```python
from build123d import *

# Parameters (mm, degrees)
F0_W     = 19
F0_H     = 19
F0_W_2   = 13.5
F0_H_2   = 13.5
F1_DEPTH = 12.5
F2_W     = 25
F2_H     = 34
F3_DEPTH = 2.5
F4_W     = 25
F4_H     = 2
F5_DEPTH = 30
F6_W     = 2
F6_H     = 25
F7_DEPTH = 20
F8_W     = 32.5
F8_H     = 10
F9_DEPTH = 2


with BuildPart() as f1:
    # F0 (on Front) → F1 (new body, symmetric)
    with BuildSketch(Plane.XZ):
        Rectangle(F0_W, F0_H)
        Rectangle(F0_W_2, F0_H_2, mode=Mode.SUBTRACT)
    extrude(amount=F1_DEPTH, both=True)

    # F2 (on face) → F3 (join)
    with BuildSketch(Plane(origin=(-9.5, 0, 0), x_dir=(0, -1, 0), z_dir=(-1, 0, 0))):
        with Locations((0, -7.5)):
            Rectangle(F2_W, F2_H)
    extrude(amount=-F3_DEPTH)

    # F4 (on face) → F5 (join)
    with BuildSketch(Plane(origin=(-9.5, 0, 0), x_dir=(0, -1, 0), z_dir=(-1, 0, 0))):
        with Locations((0, -23.5)):
            Rectangle(F4_W, F4_H)
    extrude(amount=F5_DEPTH)

    # F6 (on face) → F7 (join)
    with BuildSketch(Plane.XY.offset(-22.5)):
        with Locations((-38.5, 0)):
            Rectangle(F6_W, F6_H)
    extrude(amount=F7_DEPTH)

    # F8 (on face) → F9 (join)
    with BuildSketch(Plane(origin=(0, 12.5, 0), x_dir=(-1, 0, 0), z_dir=(0, 1, 0))):
        with Locations((23.25, -19.5)):
            Rectangle(F8_W, F8_H)
    extrude(amount=-F9_DEPTH)


solid = f1.part
```
Design review of the part built by this model. Coordinates are the model's own, in mm. A direction names the side the tool comes from. Coordinates: 2 decimals unless noted, no trailing zeros. Order: outer loops, then holes, each group sorted by start corner. A loop starts at its lowest first (then second) coordinate and runs counter-clockwise, first axis right, second up. Notation, with made-up numbers: (34, 20.25) - (41, 20.25) arc R34 ccw to (41, 58.25) - close; hole circle Ø1 at (-17, 41.25). An arc over 180 degrees is marked (long way). One line per question, with ' | ' between items.
Q1. To check wall thickness, follow line 1 along X through (y, z) = (-7.25, -5); line 2 along X through (y, z) = (8, -18); line 3 along X through (y, z) = (-10.75, -2). State the ranges of each line that lie inside material, in increasing order.
Answer key:
line 1: x = -39.5 to -37.5, -9.5 to -6.75, 6.75 to 9.5 | line 2: x = -39.5 to -37.5, -9.5 to -7 | line 3: x = -9.5 to -6.75, 6.75 to 9.5
Q2. For faces 1 (the flat face through (6.75, 0, 0)), 2 (the flat face through (-23, 12, -14.5)), 3 (the flat face through (-23, -1, -22.5)), 4 (the flat face through (-39, 0, -2.5)), 5 (the flat face through (1, 0, -9.5)), list the 3-axis set-ups (+Z, -Z, +X, -X, +Y, -Y) from which the entire face can be reached by the end or side of a thin tool; tool diameter is ignored.
Answer key:
face 1: +Y, -Y | face 2: +Z, +Y, -Y | face 3: +Z, -Y | face 4: +Z, -X, +Y, -Y | face 5: -Z, +X, +Y, -Y
Q3. Consider section C-C, the plane y = 0.75. Give the boundary of the cut face in (x, z), then the cut area to 3 significant figures.
Answer key:
outline: (-39.5, -24.5) - (-7, -24.5) - (-7, -9.5) - (9.5, -9.5) - (9.5, 9.5) - (-9.5, 9.5) - (-9.5, -22.5) - (-37.5, -22.5) - (-37.5, -2.5) - (-39.5, -2.5) - close; hole (-6.75, -6.75) - (6.75, -6.75) - (6.75, 6.75) - (-6.75, 6.75) - close | area: 316 mm2
Q4. Consider section A-A, the plane z = -1. Give the boundary of the cut face in (x, y), then the cut area to 4 significant figures.
Answer key:
outline: (-9.5, -12.5) - (-6.75, -12.5) - (-6.75, 12.5) - (-9.5, 12.5) - close; (6.75, -12.5) - (9.5, -12.5) - (9.5, 12.5) - (6.75, 12.5) - close | area: 137.5 mm2
Q5. Clearance check with flat-ended pins moving along their axes: pin 1 Ø8 at (y, z) = (0.5, 0) entering from -X; pin 2 Ø11.5 at (x, y) = (-20, -5.5) entering from +Z; pin 3 Ø6 at (x, y) = (2, -8.5) entering from -Z; pin 4 Ø12 at (x, z) = (-27.5, -3.5) entering from -Y. State where each tip first meets the part, or that it passes through.
Answer key:
pin 1: stops at x = -39.5 | pin 2: stops at z = -22.5 | pin 3: stops at z = -9.5 | pin 4: passes through
Q6. Consider section B-B, the plane x = 1.5. Give the boundary of the cut face in (y, z).
Answer key:
outline: (-12.5, -9.5) - (12.5, -9.5) - (12.5, -6.75) - (-12.5, -6.75) - close; (-12.5, 6.75) - (12.5, 6.75) - (12.5, 9.5) - (-12.5, 9.5) - close
Q7. The part is to be moulded in two halves that separate along X. For faces 6 (the flat face through (0, 0, -6.75)), 7 (the flat face through (9.5, 0, 0)), 8 (the flat face through (-19, 12.5, -15)), say which applies: +X half, -X half, draft (parallel to the pull), parting line (faces both ways), or undercut.
Answer key:
face 6: undercut | face 7: +X half | face 8: draft
Q8. Consider section D-D, the plane z = -19. Give the boundary of the cut face in (x, y).
Answer key:
outline: (-39.5, -12.5) - (-37.5, -12.5) - (-37.5, 10.5) - (-9.5, 10.5) - (-9.5, -12.5) - (-7, -12.5) - (-7, 12.5) - (-39.5, 12.5) - close
